Part model, mm, in its own coordinate system. A direction names the side the tool comes from. Round coordinates to 2 decimals unless told otherwise and drop trailing zeros. Order: outer loops, then holes, each group sorted by start corner. A loop starts at its lowest first (then second) coordinate and runs counter-clockwise, first axis right, second up. Notation, with made-up numbers: (-13.5, -21.5) - (4.5, -21.5) arc R13 cw to (4.5, 1.5) - close; hole circle Ø11 at (82.25, 79.5). An arc over 180 degrees is marked (long way). Answer as a JSON object with one key per item and string values.
```python
from build123d import *

# Parameters (mm, degrees)
BOSS_EXTRUDE2_DEPTH = 110
SKETCH3_W           = 9.744334313
SKETCH3_H           = 110
BOSS_EXTRUDE3_DEPTH = 30.2


with BuildPart() as part:
    # Sketch1 → Boss-Extrude2 (new body)
    with BuildSketch(Plane.XY):
        Polygon((0, 0), (10, 0), (10, 30), (597.2, 30), (597.2, 0), (607.2, 0), (607.2, 44.8), (0, 44.8), align=None)
    extrude(amount=BOSS_EXTRUDE2_DEPTH)

    # Sketch3 → Boss-Extrude3 (add)
    with BuildSketch(Plane(origin=(0, 39.6, 0), x_dir=(1, 0, 0), z_dir=(0, 1, 0))):
        with Locations((343.727832843, -55)):
            Rectangle(SKETCH3_W, SKETCH3_H)
        with Locations((263.472167157, -55)):
            Rectangle(SKETCH3_W, SKETCH3_H)
    extrude(amount=BOSS_EXTRUDE3_DEPTH)


solid = part.part
```
Item 1: Probe L1, parallel to X at y = 28.5, z = 63; L2, parallel to X at y = 66, z = 26.5; L3, parallel to Y at x = 89, z = 62.5. List the from-to ranges inside material, lowest first. Write a range as from..to.
Taken from the geometry:
{"L1": "0..10, 597.2..607.2", "L2": "258.6..268.34, 338.86..348.6", "L3": "30..44.8"}
Item 2: Cut at A-A (y = 64). Write the cut outline in (x, z), plus the area to 3 significant figures.
Taken from the geometry:
{"outline": "(258.6, 0) - (268.34, 0) - (268.34, 110) - (258.6, 110) - close; (338.86, 0) - (348.6, 0) - (348.6, 110) - (338.86, 110) - close", "area": "2,140 mm2"}
Item 3: Cut at B-B (z = 39.5). Write the cut outline in (x, y), plus the area to 3 significant figures.
Taken from the geometry:
{"outline": "(0, 0) - (10, 0) - (10, 30) - (597.2, 30) - (597.2, 0) - (607.2, 0) - (607.2, 44.8) - (348.6, 44.8) - (348.6, 69.8) - (338.86, 69.8) - (338.86, 44.8) - (268.34, 44.8) - (268.34, 69.8) - (258.6, 69.8) - (258.6, 44.8) - (0, 44.8) - close", "area": "10,100 mm2"}
Item 4: Two-plate mould, pull along X, no slides. Class faces 1 (the flat face through (258.6, 57, 56)), 2 (the flat face through (299, 30, 54)), 3 (the flat face through (344, 69.8, 54)): pulls with the +X half, pulls with the -X half, needs draft (parallel to the pull), parting line crosses it, or undercut.
Taken from the geometry:
{"face 1": "pulls with the -X half", "face 2": "undercut", "face 3": "needs draft"}
Item 5: Cut at C-C (y = 6). Write the cut outline in (x, z).
Taken from the geometry:
{"outline": "(0, 0) - (10, 0) - (10, 110) - (0, 110) - close; (597.2, 0) - (607.2, 0) - (607.2, 110) - (597.2, 110) - close"}
Item 6: Drop flat-ended pins along their axis: P1, Ø4, axis at y = 20.5, z = 40.5, coming from the -X side; P2, Ø12, axis at y = 56.5, z = 95, coming from the +X side; P3, Ø20, axis at y = 58.5, z = 78.5, coming from the -X side; P4, Ø21, axis at x = 298, z = 73, coming from the +Y side. Give the stop position or say it passes through.
Taken from the geometry:
{"P1": "x = 0", "P2": "x = 348.6", "P3": "x = 258.6", "P4": "y = 44.8"}
Item 7: Cut at D-D (x = 42). Write the cut outline in (y, z), plus the area to 3 significant figures.
Taken from the geometry:
{"outline": "(30, 0) - (44.8, 0) - (44.8, 110) - (30, 110) - close", "area": "1,630 mm2"}
Item 8: Tool access for faces 4 (the flat face through (480, 44.8, 54)), 5 (the flat face through (10, 15, 54)), 6 (the flat face through (304, 44.8, 54)), 7 (the flat face through (131, 44.8, 54)), 8 (the flat face through (607.2, 22, 54)): list every direction of +Z, -Z, +X, -X, +Y, -Y with a clear straight run to the whole face (end or side of a thin tool).
Taken from the geometry:
{"face 4": "+Z, -Z, +X, +Y", "face 5": "+Z, -Z, -Y", "face 6": "+Z, -Z, +Y", "face 7": "+Z, -Z, -X, +Y", "face 8": "+Z, -Z, +X, +Y, -Y"}
